from build123d import *

# Parameters (mm, degrees)
REVOLVE1_ANGLE     = 180
FILLET1_ANGLE      = 180
FILLET1_2_ANGLE    = 180
SKETCH2_W          = 2
SKETCH2_H          = 0.8
CUT_EXTRUDE1_DEPTH = 1


with BuildPart() as part:
    # Sketch1 → Revolve1 (revolve)
    with BuildSketch(Plane(origin=(0, 0, 0), x_dir=(1, 0, 0), z_dir=(0, 1, 0))):
        with BuildLine():
            Line((0, 0), (-70, 0))
            Line((-70, 0), (-70, 0.8))
            Line((-70, 0.8), (-69.8, 0.8))
            Line((-69.8, 0.8), (-62.8, 3))
            Line((-62.8, 3), (-14, 3))
            ThreePointArc((-14, 3), (-13, 2), (-12, 3))
            Line((-12, 3), (-10, 3))
            ThreePointArc((-10, 3), (-9, 2), (-8, 3))
            Line((-8, 3), (-6, 3))
            ThreePointArc((-6, 3), (-5, 2), (-4, 3))
            Line((-4, 3), (-1.5, 3))
            ThreePointArc((-1.5, 3), (-0.439339828, 2.560660172), (0, 1.5))
            Line((0, 1.5), (0, 0))
        make_face()
    revolve(axis=Axis((0, 0, 0), (1, 0, 0)), revolution_arc=REVOLVE1_ANGLE)

    # Fillet1: read off the stored shape, not the designer's step
    # Fillet1 outline → Fillet1 (revolve)
    with BuildSketch(Plane(origin=(0, 0, 0), x_dir=(0, 0, -1), z_dir=(0, -1, 0))):
        with BuildLine():
            Line((0.8, -69.518311709), (0.8, -70))
            ThreePointArc((0.8, -70), (0.829465257, -69.75643572), (0.888530606, -69.518311709))
            Line((0.888530606, -69.518311709), (0.8, -69.518311709))
        make_face()
    revolve(axis=Axis((0, 0, 0), (1, 0, 0)), revolution_arc=FILLET1_ANGLE)

    # Fillet1 2 outline → Fillet1 2 (revolve, cut)
    with BuildSketch(Plane(origin=(0, 0, 0), x_dir=(0, 0, -1), z_dir=(0, -1, 0))):
        with BuildLine():
            ThreePointArc((3, -62.493114063), (2.976863029, -62.796449795), (2.907987434, -63.092767256))
            Line((2.907987434, -63.092767256), (3, -63.092767256))
            Line((3, -63.092767256), (3, -62.493114063))
        make_face()
        with BuildLine():
            Line((3, -15.236067977), (3, -13.745355992))
            Line((3, -13.745355992), (2.333333333, -13.745355992))
            ThreePointArc((2.333333333, -13.745355992), (2.825741858, -14.419571396), (3, -15.236067977))
        make_face()
        with BuildLine():
            Line((2.333333333, -12.254644008), (3, -12.254644008))
            Line((3, -12.254644008), (3, -9.745355992))
            Line((3, -9.745355992), (2.333333333, -9.745355992))
            ThreePointArc((2.333333333, -9.745355992), (2.774276771, -10.313060967), (2.986019111, -11))
            ThreePointArc((2.986019111, -11), (2.774276771, -11.686939033), (2.333333333, -12.254644008))
        make_face()
        with BuildLine():
            Line((2.333333333, -8.254644008), (3, -8.254644008))
            Line((3, -8.254644008), (3, -5.745355992))
            Line((3, -5.745355992), (2.333333333, -5.745355992))
            ThreePointArc((2.333333333, -5.745355992), (2.774276771, -6.313060967), (2.986019111, -7))
            ThreePointArc((2.986019111, -7), (2.774276771, -7.686939033), (2.333333333, -8.254644008))
        make_face()
        with BuildLine():
            Line((2.333333333, -4.254644008), (3, -4.254644008))
            Line((3, -4.254644008), (3, -2.763932023))
            ThreePointArc((3, -2.763932023), (2.825741858, -3.580428604), (2.333333333, -4.254644008))
        make_face()
    revolve(axis=Axis((0, 0, 0), (1, 0, 0)), revolution_arc=FILLET1_2_ANGLE, mode=Mode.SUBTRACT)

    # Sketch2 → Cut-Extrude1 (cut)
    with BuildSketch(Plane.XZ):
        with Locations((-56.493114063, -2.6)):
            Rectangle(SKETCH2_W, SKETCH2_H)
        with Locations((-21.236067977, -2.6)):
            Rectangle(SKETCH2_W, SKETCH2_H)
        with Locations((-21.236067977, 2.6)):
            Rectangle(SKETCH2_W, SKETCH2_H)
        with Locations((-56.493114063, 2.6)):
            Rectangle(SKETCH2_W, SKETCH2_H)
    extrude(amount=-CUT_EXTRUDE1_DEPTH, mode=Mode.SUBTRACT)


solid = part.part
The model under review builds one solid part; all positions refer to its coordinate system, in mm. Coordinates: 2 decimals unless noted, no trailing zeros. Write each loop counter-clockwise with the first axis right and the second up, starting at its lowest first coordinate (ties: lowest second). Pieces come first, ordered by that corner, then holes. Notation, with made-up numbers: (75.25, 30.5) - (117.25, 30.5) arc R24 cw to (117.25, 62.5) - close; hole circle Ø6 at (-7, 43). An arc over 180 degrees is marked (long way). Answer as CSV lines item,"result".
(1) Clearance check with flat-ended pins moving along their axes: pin 1 Ø0.9 at (y, z) = (0.5, -2.5) entering from +X (3 decimals); pin 2 Ø0.5 at (x, y) = (-57, 0.5) entering from -Z; pin 3 Ø0.5 at (x, y) = (-21, 0.5) entering from +Z; pin 4 Ø0.7 at (x, z) = (-56.5, -2.5) entering from -Y. State where each tip first meets the part, or that it passes through.
Data:
pin 1,"stops at x = -0.125"
pin 2,"stops at z = -2.2"
pin 3,"stops at z = 2.2"
pin 4,"stops at y = 0"
(2) We need section A-A (x = -9). Give the boundary of the cut face in (y, z), plus the area to 3 significant figures.
Data:
outline,"(0, -2) arc R2 ccw to (0, 2) - close"
area,"6.28 mm2"
(3) For line 1 along X through (y, z) = (1.8, -2); line 2 along Z through (x, y) = (-57, 0.4); line 3 along Y through (x, z) = (-50, -0.25), list the stretches that pass through material, from the lowest coordinate up. Write a range as [from, to].
Data:
line 1,"x = [-63.78, -14.17], [-11.83, -10.17], [-7.83, -6.17], [-3.83, -0.59]"
line 2,"z = [-2.2, 2.2]"
line 3,"y = [0, 2.99]"
(4) We need section B-B (x = -46.5). Give the boundary of the cut face in (y, z), plus the area to 3 significant figures.
Data:
outline,"(0, -3) arc R3 ccw to (0, 3) - close"
area,"14.1 mm2"
